Design review of the part built by this model. Coordinates are the model's own, in mm. A direction names the side the tool comes from. Coordinates: 2 decimals unless noted, no trailing zeros. Loops run counter-clockwise (first coordinate to the right, second up) from the corner with the lowest first, then second, coordinate; pieces in that order, holes last. Notation, with made-up numbers: (49, 89) -> (73, 89) arc R35 ccw to (73, 127) -> close; hole circle Ø4 at (-4, 5). An arc over 180 degrees is marked (long way). One line per item, written item: value. Start each with the question number.
1. Insertion check: pin 1 (6.5 mm diameter, centred on x = 1, y = -5, fed in from +Z); pin 2 (5 mm diameter, centred on x = -2.5, y = -7, fed in from -Z); pin 3 (6 mm diameter, centred on x = -8, z = 2.5, fed in from +Y); pin 4 (6.5 mm diameter, centred on x = -9.5, y = -50, fed in from -Z). Each pin has a flat end and moves straight along its axis. Give the tip position at first contact, or say it passes through.
2. Draft analysis for pull direction Y (two halves, no side actions). For faces 4 (the flat face through (-9.542, -55.646, 17.321)), 5 (the cylindrical face through (-12.07, -51.33, -7.8)), 6 (the cylindrical face through (-12.07, -23.54, -24.55)), state which applies: pulls with the +Y half, pulls with the -Y half, needs draft (parallel to the pull), parting line crosses it, or undercut.
3. For probe 1 along X at (y, z) = (0, -21.8); probe 2 along X at (y, z) = (-42, 0.5); probe 3 along Z at (x, y) = (3, -20), list the stretches that pass through material, from the lowest coordinate up.
4. Add section B-B on y = -21. Write out the cut boundary in (x, z), plus the area to 3 significant figures.
5. Machinability: for faces 1 (the cylindrical face through (12.05, -23.54, -24.57)), 2 (the cylindrical face through (12.07, -16.22, -0.45)), 3 (the flat face through (-10, -50, 20.55)), which of the approach directions +Z, -Z, +X, -X, +Y, -Y give a long, thin tool a straight path to every point of the face, cutting with its end or side? Answer none if there is none.
6. Add section A-A on x = 0. Give the number of separate pieces and of enclosed holes in the cut face, plus the area to 3 significant figures.
Autodesk Inventor part; units mm, degrees
ref_plane "YZ Plane" through (0, 0, 0) normal (1, 0, 0) x (0, 1, 0)
ref_plane "XZ Plane" through (0, 0, 0) normal (0, 1, 0) x (-1, 0, 0)
ref_plane "XY Plane" through (0, 0, 0) normal (0, 0, 1) x (1, 0, 0)
sketch "Sketch1" plane through (0, 0, 0) normal (1, 0, 0) x (0, 1, 0)
  circle A0 centre (-50, 14) radius 4.05
  arc A1 (-39.1747, 20.25) -> (-60.8253, 7.75) centre (-50, 14) ccw
  line L0 (0, 0) -> (0, -25)
  line L1 (0, -25) -> (-41.9171, -25)
  line L2 (-41.9171, -25) -> (-60.8253, 7.75)
  line L3 (0, 0) -> (-27.4833, 0)
  line L4 (-27.4833, 0) -> (-39.1747, 20.25)
  dimension "d0" = 8.1
  dimension "d2" = 50
  dimension "d3" = 14
  dimension "d4" = 25
  dimension "d6" = 25
  dimension "d40" = 120
extrude "Extrusion1" add sketch "Sketch1" along normal mid plane 25
sketch "Sketch2" plane through (-12.5, -27.4833, 0) normal (0, 0, 1) x (1, 0, 0)
  circle A0 centre (12.5, 27.4833) radius 12.5
extrude "Extrusion2" add sketch "Sketch2" against normal up to surface (25 mm away)
sketch "Sketch12" plane through (-12.5, 0, 0) normal (-1, 0, 0) x (0, 0, 1)
  circle A0 centre (14, -50) radius 4.05
  arc A1 (7.75, -60.8253) -> (20.25, -39.1747) centre (14, -50) ccw
  line L0 (14, -42.4367) -> (20.55, -46.2184)
  line L1 (20.55, -46.2184) -> (20.55, -53.7816)
  line L2 (20.55, -53.7816) -> (14, -57.5633)
  line L3 (14, -57.5633) -> (7.45, -53.7816)
  line L4 (7.45, -53.7816) -> (7.45, -46.2184)
  line L5 (7.45, -46.2184) -> (14, -42.4367)
  dimension "d56" = 13.1
extrude "Extrusion12" cut sketch "Sketch12" against normal blind 6
sketch "Sketch13" plane through (-12.5, -27.4833, 0) normal (0, 0, 1) x (1, 0, 0)
  arc A0 (25, 27.4833) -> (0, 27.4833) centre (12.5, 27.4833) ccw
  circle A1 centre (12.5, 27.4833) radius 9.05
  dimension "d59" = 18.1
extrude "Extrusion13" cut sketch "Sketch13" against normal through all
sketch "Sketch14" plane through (-12.5, -27.4833, 0) normal (0, 0, 1) x (1, 0, 0)
  circle A0 centre (12.5, 27.4833) radius 9.05
  arc A1 (25, 27.4833) -> (0, 27.4833) centre (12.5, 27.4833) ccw
  circle A2 centre (12.5, 27.4833) radius 10.55
  dimension "d63" = 21.1
extrude "Extrusion14" cut sketch "Sketch14" against normal blind 4
sketch "Sketch15" plane through (12.5, -41.9171, -25) normal (0, 0, -1) x (-1, 0, 0)
  circle A0 centre (12.5, 41.9171) radius 9.05
  arc A1 (25, 41.9171) -> (0, 41.9171) centre (12.5, 41.9171) ccw
  circle A2 centre (12.5, 41.9171) radius 10.55
  dimension "d67" = 21.1
extrude "Extrusion15" cut sketch "Sketch15" against normal blind 4
chamfer "Chamfer4" distance 1.5 angle 45 1 edges at (-9.05, 0, -21)
sketch "Sketch16" plane through (-12.5, -27.4833, 0) normal (0, 0, 1) x (1, 0, 0)
  circle A0 centre (12.5, 27.4833) radius 10.55
  arc A1 (25, 27.4833) -> (0, 27.4833) centre (12.5, 27.4833) ccw
  circle A2 centre (12.5, 27.4833) radius 13.55
  dimension "d76" = 3
extrude "Extrusion16" add sketch "Sketch16" against normal up to surface (25 mm away)
fillet "Fillet2" radius 1.5 16 edges at (0, -41.9171, -25) (12.5, -51.3712, -8.625) (-12.5, -51.3712, -8.625) (12.5, -56.25, 24.8253) (12.5, -33.329, 10.125) (-12.5, -56.25, 24.8253) (-12.5, -33.329, 10.125) (12.5, -23.5735, -25) (-12.5, -23.5735, -25) (0, 13.55, -25) (-12.5, -5.23, -12.5) (0, 13.55, 0) (12.5, -5.23, -12.5) (-12.5, -16.3567, 0) (0, -27.4833, 0) (12.5, -16.3567, 0)
properties part number "hub top"
Worked answers:
1. pin 1: passes through
1. pin 2: stops at z = -20.38
1. pin 3: stops at y = 10.94
1. pin 4: stops at z = -16.63
2. face 4: undercut
2. face 5: pulls with the -Y half
2. face 6: needs draft
3. probe 1: x = -13.55 to -10.55, 10.55 to 13.55
3. probe 2: x = -12.5 to 12.5
3. probe 3: z = -25 to 0
4. outline: (-12.5, -23.5) arc R1.5 ccw to (-11, -25) -> (11, -25) arc R1.5 ccw to (12.5, -23.5) -> (12.5, -1.5) arc R1.5 ccw to (11, 0) -> (-11, 0) arc R1.5 ccw to (-12.5, -1.5) -> close
4. area: 623 mm²
5. face 1: -Z, +X, -Y
5. face 2: +Z, +X
5. face 3: -X
6. separate pieces: 2
6. enclosed holes: 1
6. area: 1,690 mm²
